```python
from build123d import *

# Parameters (mm, degrees)
F0_W      = 153.852672
F0_H      = 350.459368
F1_DEPTH  = 6.35
F2_W      = 153.852672
F2_H      = 6.35
F3_DEPTH  = 127
F4_W      = 153.852672
F4_H      = 6.35
F5_DEPTH  = 127
F7_DEPTH  = 96.774
F8_W      = 70.44766
F8_H      = 80.216594
F8_R      = 25.993866
F9_DEPTH  = 25.4
F10_W     = 27.971894
F10_H     = 93.894914
F11_DEPTH = 127


with BuildPart() as f1:
    # F0 (on Top) → F1 (new body)
    with BuildSketch(Plane.XY):
        Rectangle(F0_W, F0_H)
    extrude(amount=F1_DEPTH)

    # F2 (on face) → F3 (join)
    with BuildSketch(Plane.XY.offset(6.35)):
        with Locations((0, 130.175)):
            Rectangle(F2_W, F2_H)
    extrude(amount=F3_DEPTH)

    # F4 (on face) → F5 (join)
    with BuildSketch(Plane.XY.offset(6.35)):
        with Locations((0, 104.775)):
            Rectangle(F4_W, F4_H)
    extrude(amount=F5_DEPTH)

    # F6 (on face) → F7 (cut)
    with BuildSketch(Plane(origin=(0, 133.35, 0), x_dir=(-1, 0, 0), z_dir=(0, 1, 0))):
        with BuildLine():
            Line((12.7, 133.35), (0, 133.35))
            Line((0, 133.35), (-12.7, 133.35))
            Line((-12.7, 133.35), (-12.7, 69.85))
            ThreePointArc((-12.7, 69.85), (0, 57.15), (12.7, 69.85))
            Line((12.7, 69.85), (12.7, 133.35))
        make_face()
    extrude(amount=-F7_DEPTH, mode=Mode.SUBTRACT)

    # F8 (on face) → F9 (join)
    with BuildSketch(Plane.XY.offset(6.35)):
        Rectangle(F8_W, F8_H)
        Circle(F8_R, mode=Mode.SUBTRACT)
    extrude(amount=F9_DEPTH)

    # F10 (on face) → F11 (join)
    with BuildSketch(Plane.XY.offset(6.35)):
        with Locations((-62.940389, -128.282227)):
            Rectangle(F10_W, F10_H)
    extrude(amount=F11_DEPTH)


solid = f1.part
```
Check sheet for the modelled part. Datum: model origin and axes. Units: mm. A direction names the side the tool comes from. Round coordinates to 2 decimals unless told otherwise and drop trailing zeros. Loops run counter-clockwise (first coordinate to the right, second up) from the corner with the lowest first, then second, coordinate; pieces in that order, holes last. Notation, with made-up numbers: M 71.25,-15 L 105.25,-15 A27 cw 105.25,7 Z; hole C 69.25,2 d11. An arc over 180 degrees is marked long. Answer as a JSON object with one key per item and string values.
1. Section check A-A (z = 27). Record the boundary of the cut face in (x, y).
Reply:
{"outline": "M -76.93,-175.23 L -48.95,-175.23 L -48.95,-81.33 L -76.93,-81.33 Z; M -76.93,101.6 L 76.93,101.6 L 76.93,107.95 L -76.93,107.95 Z; M -76.93,127 L 76.93,127 L 76.93,133.35 L -76.93,133.35 Z; M -35.22,-40.11 L 35.22,-40.11 L 35.22,40.11 L -35.22,40.11 Z; hole C 0,0 d51.99"}
2. Gauge pin test, flat ends, axial feed: P1, Ø21, axis at x = 16, y = -7, coming from the +Z side; P2, Ø12, axis at x = 11, z = 48.5, coming from the +Y side; P3, Ø5, axis at x = 12.5, z = 37.5, coming from the +Y side. Record the tip position at first contact, or that the pin passes through.
Reply:
{"P1": "stops at z = 31.75", "P2": "stops at y = 133.35", "P3": "stops at y = 133.35"}
3. Section check C-C (z = 78.5). Record the boundary of the cut face in (x, y), plus the area to 3 significant figures.
Reply:
{"outline": "M -76.93,-175.23 L -48.95,-175.23 L -48.95,-81.33 L -76.93,-81.33 Z; M -76.93,101.6 L -12.7,101.6 L -12.7,107.95 L -76.93,107.95 Z; M -76.93,127 L -12.7,127 L -12.7,133.35 L -76.93,133.35 Z; M 12.7,101.6 L 76.93,101.6 L 76.93,107.95 L 12.7,107.95 Z; M 12.7,127 L 76.93,127 L 76.93,133.35 L 12.7,133.35 Z", "area": "4,260 mm²"}
4. Access from +Z, -Z, +X, -X, +Y, -Y to the whole of each face (thin tool, end or side, straight path). Record for faces 4 (the flat face through (-12.7, 130, 101)), 5 (the flat face through (-1, 118, 6.35)), 6 (the flat face through (0, -40.108, 19)), 7 (the flat face through (-1, 155, 6.35)).
Reply:
{"face 4": "+Z, +Y, -Y", "face 5": "+Z, +X, -X", "face 6": "+Z, +X, -X, -Y", "face 7": "+Z, +X, -X, +Y"}
5. Section check B-B (x = 0). Record the boundary of the cut face in (y, z).
Reply:
{"outline": "M -175.23,0 L 175.23,0 L 175.23,6.35 L 133.35,6.35 L 133.35,57.15 L 127,57.15 L 127,6.35 L 107.95,6.35 L 107.95,57.15 L 101.6,57.15 L 101.6,6.35 L 40.11,6.35 L 40.11,31.75 L 25.99,31.75 L 25.99,6.35 L -25.99,6.35 L -25.99,31.75 L -40.11,31.75 L -40.11,6.35 L -175.23,6.35 Z"}
6. Section check D-D (y = 0). Record the boundary of the cut face in (x, z).
Reply:
{"outline": "M -76.93,0 L 76.93,0 L 76.93,6.35 L 35.22,6.35 L 35.22,31.75 L 25.99,31.75 L 25.99,6.35 L -25.99,6.35 L -25.99,31.75 L -35.22,31.75 L -35.22,6.35 L -76.93,6.35 Z"}
7. Mould release check, pull along Y, two halves, no side actions. Record for faces 1 (the flat face through (-1, 101.6, 55)), 2 (the flat face through (-1, 2, 0)), 3 (the flat face through (-52, -175.23, 61)): pulls with the +Y half, pulls with the -Y half, needs draft (parallel to the pull), parting line crosses it, or undercut.
Reply:
{"face 1": "undercut", "face 2": "needs draft", "face 3": "pulls with the -Y half"}
8. Scan lines: line 1 (Y direction, x = -66, z = 80); line 2 (Y direction, x = 0, z = 25); line 3 (Y direction, x = -45, z = 110). Record each from-to range of solid material in increasing order.
Reply:
{"line 1": "y = -175.23 to -81.33, 101.6 to 107.95, 127 to 133.35", "line 2": "y = -40.11 to -25.99, 25.99 to 40.11, 101.6 to 107.95, 127 to 133.35", "line 3": "y = 101.6 to 107.95, 127 to 133.35"}
